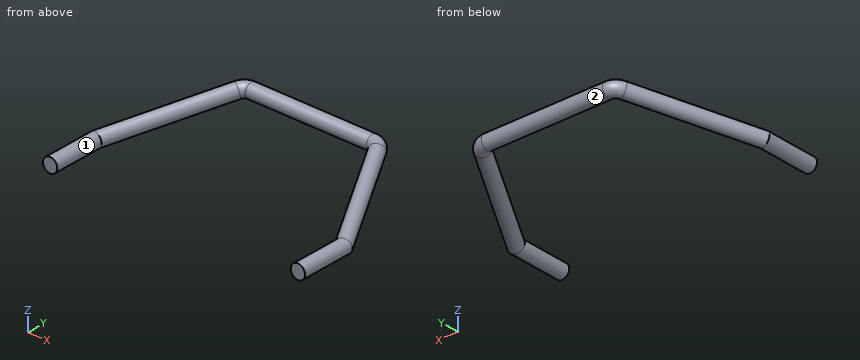
from build123d import *

# Parameters (mm, degrees)
CROQUIS2_R = 3.25


with BuildPart() as part:
    # Barrer2: sweep along a curve in space
    with BuildLine() as barrer2_path:
        Line((-27.572352062, 71.613970134, 9.809651149), (0, 71.613970134, 9.809651149))
        ThreePointArc((-31.991027423, 69.008310978, 9.274420134), (-30.151141692, 70.912292174, 9.665518788), (-27.572352062, 71.613970134, 9.809651149))
        Line((-56.4, 23.857755349, 0), (-31.991027423, 69.008310978, 9.274420134))
        Line((-56.4, 0, 0), (-56.4, 23.857755349, 0))
    # Croquis2 → Barrer2 (sweep)
    with BuildSketch(Plane(origin=(0, 0, 0), x_dir=(1, 0, 0), z_dir=(0, 1, 0))):
        with Locations((-56.4, 0)):
            Circle(CROQUIS2_R)
    barrer2 = sweep(path=barrer2_path.line, transition=Transition.RIGHT)

    # Simetría1: Barrer2 across Right Plane
    add(barrer2.mirror(Plane(origin=(0, 0, 0), x_dir=(0, 0, -1), z_dir=(1, 0, 0))))


solid = part.part
Input: part model. Units: mm. Frame: model coordinates. Face numbers are marked on the shaded views. A direction names the side the tool comes from. Round coordinates to 2 decimals unless told otherwise and drop trailing zeros. Write each loop counter-clockwise with the first axis right and the second up, starting at its lowest first coordinate (ties: lowest second). Pieces come first, ordered by that corner, then holes.
1) Cut plane A-A (x = 8.5). Return the cut outline in (y, z).
2) Contact query for flat-ended pins moving along their axis: P1, Ø6, axis at x = -32.5, z = 11, coming from the -Y side; P2, Ø3, axis at x = -45.5, z = 6.5, coming from the -Y side; P3, Ø6, axis at x = 46, z = 7, coming from the +Y side. Output: stop coordinate, or through.
3) Reachability of the marked faces 1 and 2 from +Z, -Z, +X, -X, +Y, -Y: full face, straight path, thin tool, end or side. Return the list, or none.
4) Ray query, L1, parallel to X at y = 65.5, z = 11; L2, parallel to X at y = 32.5, z = -0.75; L3, parallel to Y at x = 43.5, z = 3. Return the intervals inside material, ascending.
Geometry says:
1. outline: circle Ø6.5 at (71.61, 9.81)
2. P1: stops at y = 58.06
2. P2: stops at y = 37.42
2. P3: stops at y = 55.37
3. face 1: -Y
3. face 2: none
4. L1: x = -36.11 to -31.14, 31.14 to 36.11
4. L2: x = -54.38 to -49.61, 49.61 to 54.38
4. L3: y = 41.12 to 51.99
